Part model, mm, in its own coordinate system. Face numbers are marked on the shaded views. A direction names the side the tool comes from. Round coordinates to 2 decimals unless told otherwise and drop trailing zeros. Write each loop counter-clockwise with the first axis right and the second up, starting at its lowest first coordinate (ties: lowest second). Pieces come first, ordered by that corner, then holes.
1) Drill centre lines: L1, parallel to Y at x = 9, z = 32.5 (3 decimals); L2, parallel to X at y = 34, z = 38.05; L3, parallel to X at y = 15, z = 24.5 (3 decimals). Where is each one in solid material? Low to high.
2) Saw through at A-A on x = -1. Write the cut outline in (y, z), and give its area (3 significant figures).
3) Saw through at D-D on z = 34. Write the cut outline in (x, y) (3 decimals).
4) Saw through at C-C on z = 11.5. Write the cut outline in (x, y), and give its area (3 significant figures).
5) Which spindle directions (+Z, -Z, +X, -X, +Y, -Y) get a long thin tool onto all of the face, cutting with end or side? Do the marked faces 1, 2, 3, 4 and 5. Say none if no direction does.
6) Saw through at B-B on y = 15. Write the cut outline in (x, z) (3 decimals).
7) Pull direction Y, two halves, no side cores. Call the marked faces 6, 7 and 8: +Y half, -Y half, draft (parallel to the pull), parting line (faces both ways), or undercut.
8) Flat gauge pins, fed straight in: pin 1 (9.5 mm diameter, centred on y = 30, z = 12, fed in from +X); pin 2 (2.5 mm diameter, centred on x = -24, y = 36.5, fed in from -Z); pin 3 (3 mm diameter, centred on y = 21.5, z = 29, fed in from -X); pin 4 (9 mm diameter, centred on x = 9, y = 34, fed in from -Z). Where does each tip first touch, or does it go through?
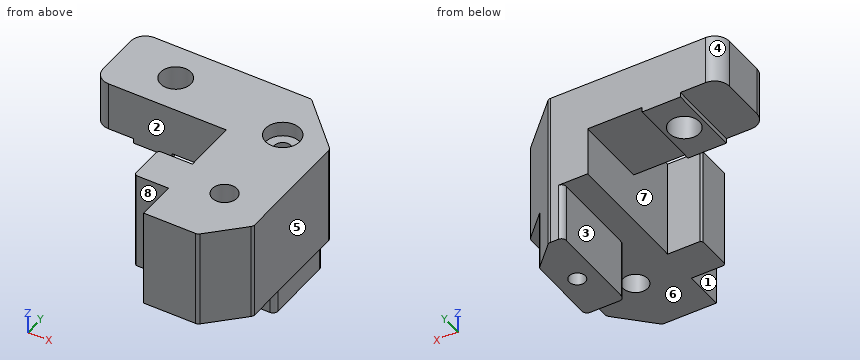
```python
from build123d import *

# Parameters (mm, degrees)
CYLINDER005_R     = 1.65
CYLINDER005_DEPTH = 40
CYLINDER001_R     = 2.525
CYLINDER001_DEPTH = 35
CYLINDER006_R     = 3.5
CYLINDER006_DEPTH = 10
CYLINDER_R        = 3.1
CYLINDER_DEPTH    = 15
BOX001_W          = 18
BOX001_H          = 42
BOX001_DEPTH      = 20
CHAMFER013_SIZE   = 7
CHAMFER016_SIZE   = 10
FILLET002_R       = 1
BOX002_W          = 7
BOX002_H          = 7.8
BOX002_DEPTH      = 20
CHAMFER011_SIZE   = 0.4
BOX015_W          = 8
BOX015_H          = 20
BOX015_DEPTH      = 12
CHAMFER009_SIZE   = 5
FILLET001_R       = 1
FILLET003_R       = 1
BOX013_W          = 7.8
BOX013_H          = 15
BOX013_DEPTH      = 1
BOX011_W          = 27
BOX011_H          = 15
BOX011_DEPTH      = 10
FILLET_R          = 3


with BuildPart() as cylinder005:
    # Cylinder005 → Cylinder005 (new body)
    with BuildSketch(Plane(origin=(9, 34, 3), x_dir=(1, 0, 0), z_dir=(0, 0, 1))):
        Circle(CYLINDER005_R)
    extrude(amount=CYLINDER005_DEPTH)


with BuildPart() as cylinder001:
    # Cylinder001 → Cylinder001 (new body)
    with BuildSketch(Plane(origin=(9, 15, 13), x_dir=(1, 0, 0), z_dir=(0, 0, 1))):
        Circle(CYLINDER001_R)
    extrude(amount=CYLINDER001_DEPTH)


with BuildPart() as cylinder006:
    # Cylinder006 → Cylinder006 (new body)
    with BuildSketch(Plane(origin=(9, 34, 37), x_dir=(1, 0, 0), z_dir=(0, 0, 1))):
        Circle(CYLINDER006_R)
    extrude(amount=CYLINDER006_DEPTH)


with BuildPart() as cylinder:
    # Cylinder → Cylinder (new body)
    with BuildSketch(Plane(origin=(-15, 37.5, 27), x_dir=(1, 0, 0), z_dir=(0, 0, 1))):
        Circle(CYLINDER_R)
    extrude(amount=CYLINDER_DEPTH)


with BuildPart() as fillet002:
    # Box001 → Box001 (new body)
    with BuildSketch(Plane(origin=(0, 3, 20), x_dir=(1, 0, 0), z_dir=(0, 0, 1))):
        with Locations((9, 21)):
            Rectangle(BOX001_W, BOX001_H)
    extrude(amount=BOX001_DEPTH)

    # Chamfer013
    chamfer013_edges = [fillet002.edges().sort_by_distance(p)[0] for p in [
        (18, 3, 30),
    ]]
    chamfer(chamfer013_edges, length=CHAMFER013_SIZE)

    # Chamfer016
    chamfer016_edges = [fillet002.edges().sort_by_distance(p)[0] for p in [
        (18, 45, 30),
    ]]
    chamfer(chamfer016_edges, length=CHAMFER016_SIZE)

    # Fillet002
    fillet002_edges = [fillet002.edges().sort_by_distance(p)[0] for p in [
        (18, 35, 30),
        (18, 10, 30),
        (8, 45, 30),
        (11, 3, 30),
    ]]
    fillet(fillet002_edges, radius=FILLET002_R)


with BuildPart() as chamfer011:
    # Box002 → Box002 (new body)
    with BuildSketch(Plane(origin=(-7, 11.1, 20), x_dir=(1, 0, 0), z_dir=(0, 0, 1))):
        with Locations((3.5, 3.9)):
            Rectangle(BOX002_W, BOX002_H)
    extrude(amount=BOX002_DEPTH)

    # Chamfer011
    chamfer011_edges = [chamfer011.edges().sort_by_distance(p)[0] for p in [
        (-7, 11.1, 30),
        (-7, 18.9, 30),
    ]]
    chamfer(chamfer011_edges, length=CHAMFER011_SIZE)


with BuildPart() as fillet003:
    # Box015 → Box015 (new body)
    with BuildSketch(Plane(origin=(7, 25, 8), x_dir=(1, 0, 0), z_dir=(0, 0, 1))):
        with Locations((4, 10)):
            Rectangle(BOX015_W, BOX015_H)
    extrude(amount=BOX015_DEPTH)

    # Chamfer009
    chamfer009_edges = [fillet003.edges().sort_by_distance(p)[0] for p in [
        (15, 45, 14),
    ]]
    chamfer(chamfer009_edges, length=CHAMFER009_SIZE)

    # Fillet001
    fillet001_edges = [fillet003.edges().sort_by_distance(p)[0] for p in [
        (15, 40, 14),
        (15, 25, 14),
        (7, 25, 14),
        (7, 45, 14),
    ]]
    fillet(fillet001_edges, radius=FILLET001_R)


with BuildPart() as fillet003_1:
    # Fillet001 placement: moved
    add(fillet003.part.moved(Location((-2, 0, 0))))

    # Fillet003
    fillet003_edges = [fillet003_1.edges().sort_by_distance(p)[0] for p in [
        (8, 45, 14),
    ]]
    fillet(fillet003_edges, radius=FILLET003_R)


with BuildPart() as cube013:
    # Box013 → Box013 (new body)
    with BuildSketch(Plane(origin=(-18.9, 30, 29), x_dir=(1, 0, 0), z_dir=(0, 0, 1))):
        with Locations((3.9, 7.5)):
            Rectangle(BOX013_W, BOX013_H)
    extrude(amount=BOX013_DEPTH)


with BuildPart() as cut002002002007004:
    # Box011 → Box011 (new body)
    with BuildSketch(Plane(origin=(-27, 30, 30), x_dir=(1, 0, 0), z_dir=(0, 0, 1))):
        with Locations((13.5, 7.5)):
            Rectangle(BOX011_W, BOX011_H)
    extrude(amount=BOX011_DEPTH)

    # Fillet
    fillet_edges = [cut002002002007004.edges().sort_by_distance(p)[0] for p in [
        (-27, 30, 35),
        (-27, 45, 35),
    ]]
    fillet(fillet_edges, radius=FILLET_R)

    # Fusion: union Cube013
    add(cube013.part)

    # Fusion006004: union Fillet002, Chamfer011, Fillet003
    add(fillet002.part)
    add(chamfer011.part)
    add(fillet003_1.part)

    # Cut: cut Cylinder
    add(cylinder.part, mode=Mode.SUBTRACT)

    # Cut002002002007002: cut Cylinder006
    add(cylinder006.part, mode=Mode.SUBTRACT)

    # Cut002002002007003: cut Cylinder001
    add(cylinder001.part, mode=Mode.SUBTRACT)

    # Cut002002002007004: cut Cylinder005
    add(cylinder005.part, mode=Mode.SUBTRACT)


solid = cut002002002007004.part
```
Completed:
1. L1: y = 3 to 12.475, 17.525 to 32.35, 35.65 to 44
1. L2: x = -27 to 5.5, 12.5 to 18
1. L3: x = -7 to 6.475, 11.525 to 18
2. outline: (11.1, 20) - (18.9, 20) - (18.9, 40) - (11.1, 40) - close; (30, 30) - (45, 30) - (45, 40) - (30, 40) - close
2. area: 306 mm2
3. outline: (-27, 33) arc R3 ccw to (-24, 30) - (0, 30) - (0, 18.9) - (-6.6, 18.9) - (-7, 18.5) - (-7, 11.5) - (-6.6, 11.1) - (0, 11.1) - (0, 3) - (10.586, 3) arc R1 ccw to (11.293, 3.293) - (17.707, 9.707) arc R1 ccw to (18, 10.414) - (18, 34.586) arc R1 ccw to (17.707, 35.293) - (8.293, 44.707) arc R1 ccw to (7.586, 45) - (-24, 45) arc R3 ccw to (-27, 42) - close; hole circle Ø6.2 at (-15, 37.5); hole circle Ø5.05 at (9, 15); hole circle Ø3.3 at (9, 34)
4. outline: (5, 26) arc R1 ccw to (6, 25) - (12, 25) arc R1 ccw to (13, 26) - (13, 39.59) arc R1 ccw to (12.71, 40.29) - (8.29, 44.71) arc R1 ccw to (7.59, 45) - (6, 45) arc R1 ccw to (5, 44) - close; hole circle Ø3.3 at (9, 34)
4. area: 138 mm2
5. face 1: +Z, -Z, -X, -Y
5. face 2: +Z, -Z, -X
5. face 3: -Z, -X, +Y, -Y
5. face 4: +Z, -Z, -X, +Y
5. face 5: +Z, -Z, +X, +Y, -Y
6. outline: (-7, 20) - (6.475, 20) - (6.475, 40) - (-7, 40) - close; (11.525, 20) - (18, 20) - (18, 40) - (11.525, 40) - close
7. face 6: draft
7. face 7: undercut
7. face 8: -Y half
8. pin 1: stops at x = 13
8. pin 2: stops at z = 30
8. pin 3: stops at x = 0
8. pin 4: stops at z = 8
